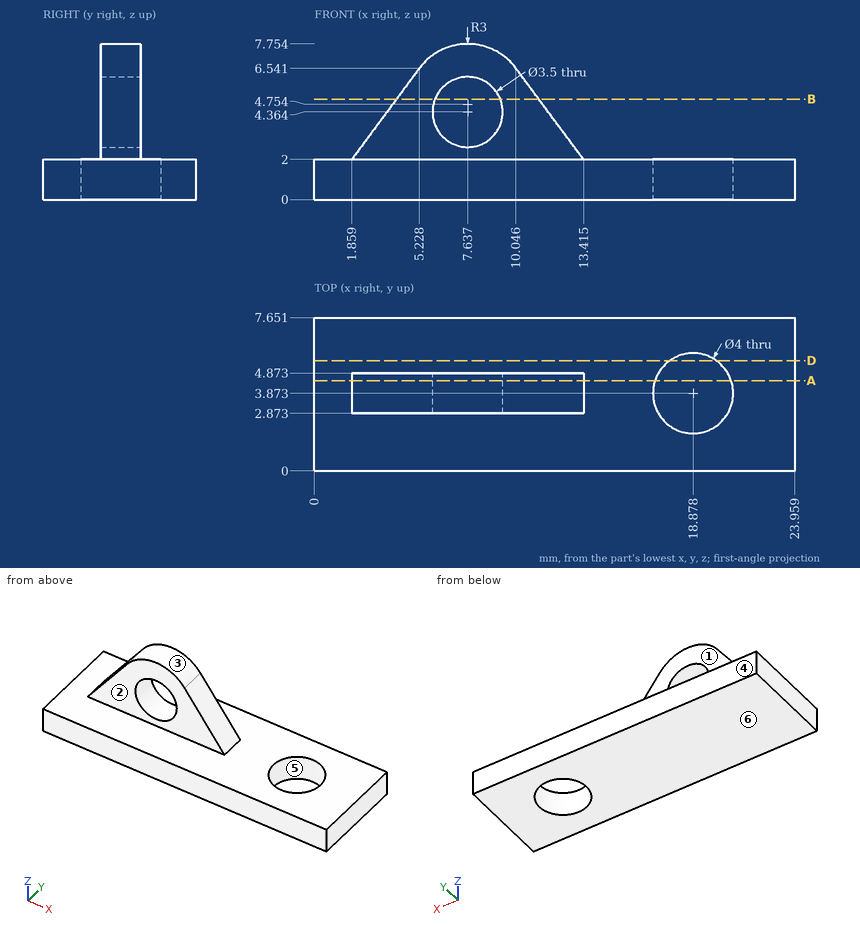
Source: three-view drawing plus pictorial views. Frame: mm from the lowest corner of the part. A direction names the side the tool comes from. Round coordinates to 2 decimals unless told otherwise and drop trailing zeros. Write each loop counter-clockwise with the first axis right and the second up, starting at its lowest first coordinate (ties: lowest second). Pieces come first, ordered by that corner, then holes. Notation, with made-up numbers: M 87,10.25 L 127,10.25 A25 cw 127,22.25 Z; hole C 11,74.25 d8. An arc over 180 degrees is marked long. One line per item, written item: value. Start each with the question number.
Item 1: Section query A-A (y = 4.5). State how many separate pieces and enclosed holes the cut face has.
Item 2: Pin query (flat end, axial travel): pin 1 (3 mm diameter, centred on x = 7.5, z = 5, fed in from -Y); pin 2 (3 mm diameter, centred on y = 6, z = 4, fed in from +X) (1 decimal). Return the tip coordinate at first contact, or that it passes through.
Item 3: Section query D-D (y = 5.5). Return the cut outline in (x, z) (1 decimal).
Item 4: Ray query, L1, parallel to Z at x = 7.75, y = 3.5; L2, parallel to Y at x = 11, z = 3.5; L3, parallel to Z at x = 16.5, y = 1.5. Return the intervals inside material, ascending. Write a range as from..to.
Item 5: Set-up query: the marked faces 1, 2 and 3. Return all of +Z, -Z, +X, -X, +Y, -Y with unobstructed straight access to the full face (end or side cutting, diameter ignored); none if empty.
Item 6: Mould query, pull axis Y, two halves, no side actions, for the marked faces 4, 5 and 6. Classes: pulls with the +Y half, pulls with the -Y half, needs draft (parallel to the pull), parting line crosses it, or undercut.
Item 7: Section query B-B (z = 5). Return the cut outline in (x, y) (1 decimal).
Result set:
1. separate pieces: 2
1. enclosed holes: 1
2. pin 1: stops at y = 2.87
2. pin 2: stops at x = 12.7
3. outline: M 0,0 L 17.7,0 L 17.7,2 L 0,2 Z; M 20,0 L 24,0 L 24,2 L 20,2 Z
4. L1: z = 0..2.62, 6.11..7.75
4. L2: y = 2.87..4.87
4. L3: z = 0..2
5. face 1: +Z, +X, -X, +Y
5. face 2: +Z, +X, -X, -Y
5. face 3: +Z, +Y, -Y
6. face 4: pulls with the +Y half
6. face 5: undercut
6. face 6: needs draft
7. outline: M 4.1,2.9 L 6,2.9 L 6,4.9 L 4.1,4.9 Z; M 9.3,2.9 L 11.2,2.9 L 11.2,4.9 L 9.3,4.9 Z
